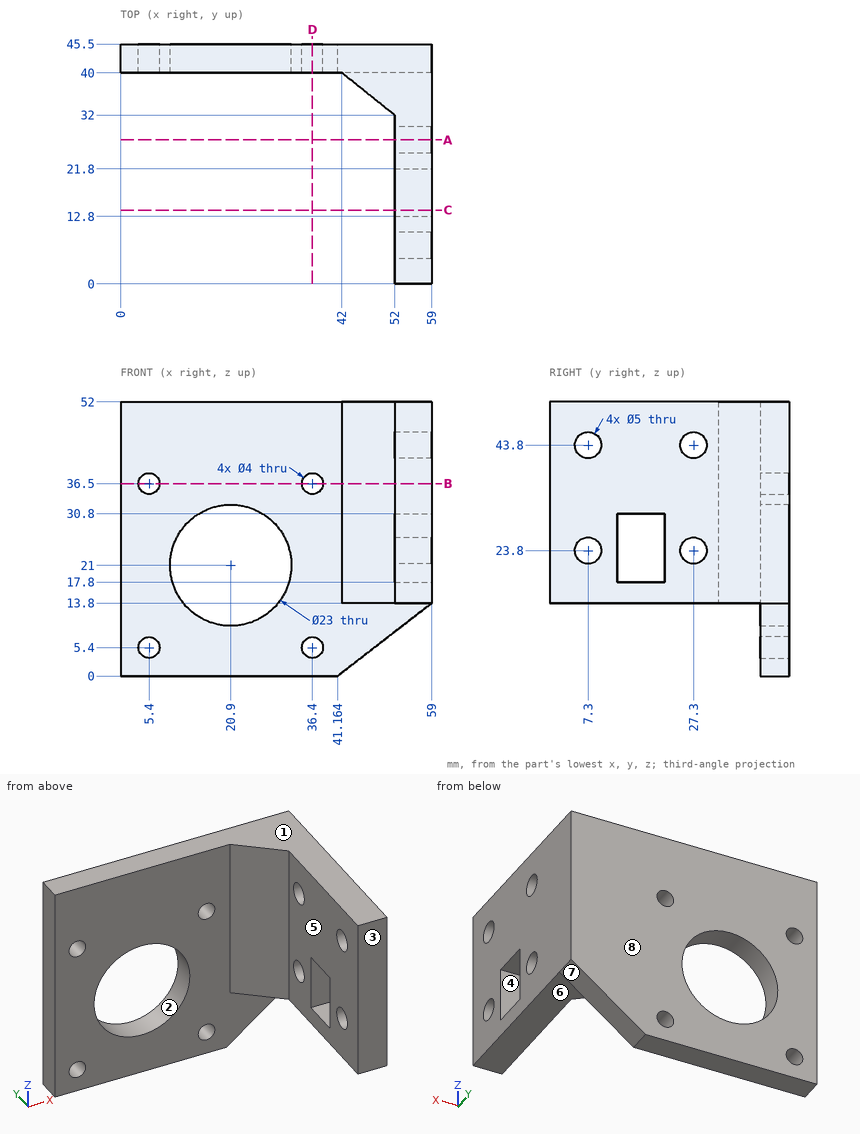
Study the drawing (mm; zero at the part's minimum x, y, z) and answer. A direction names the side the tool comes from. Coordinates: 2 decimals unless noted, no trailing zeros. Write each loop counter-clockwise with the first axis right and the second up, starting at its lowest first coordinate (ties: lowest second). Pieces come first, ordered by that corner, then holes.
Q1. Find the intervals of material crossed by line 1 (Z direction, x = 53, y = 7); line 2 (Y direction, x = 57, z = 43); line 3 (Y direction, x = 57.25, z = 43.8), in increasing order.
Q2. Which of the six approach directions +Z, -Z, +X, -X, +Y, -Y give full straight-line access (tool end or side, diameter ignored) to the marked faces 4, 5, 6, 7 and 8?
Q3. Determine the mould class of the marked faces 1, 2 and 3 for opening direction Z: released by +Z, released by -Z, zero draft, split by the parting line, or undercut.
Q4. A cutting plane is placed at B-B, the plane z = 36.5. Give the vertices of the cut face in (x, y).
Q5. A cutting plane is placed at C-C, the plane y = 14. Give the vertices of the cut face in (x, z), then the cut area to 3 significant figures.
Q6. A cutting plane is placed at D-D, the plane x = 36.4. Give the vertices of the cut face in (y, z), then the cut area to 3 significant figures.
Q7. Each of these flat-tipped pins is pushed along its axis until it touches: pin 1 Ø6.5 at (y, z) = (7.3, 23.8) entering from -X; pin 2 Ø5 at (y, z) = (11, 10) entering from -X; pin 3 Ø13.5 at (x, y) = (50.5, 25.5) entering from -Z; pin 4 Ø6.5 at (x, z) = (5.4, 36.5) entering from -Y. Where does it stop, or does it pass through?
Q8. A cutting plane is placed at A-A, the plane y = 27.3. Give the vertices of the cut face in (x, z).
Findings below:
1. line 1: z = 13.8 to 21.32, 26.28 to 41.32, 46.28 to 52
1. line 2: y = 0 to 4.93, 9.67 to 24.93, 29.67 to 45.5
1. line 3: y = 0 to 4.8, 9.8 to 24.8, 29.8 to 45.5
2. face 4: +X, -X
2. face 5: +Z, -Z, -X, -Y
2. face 6: -Z, +X, -X, -Y
2. face 7: -Z, +X, +Y, -Y
2. face 8: +Z, -Z, +X, -X, +Y
3. face 1: released by +Z
3. face 2: undercut
3. face 3: zero draft
4. outline: (0, 40) - (3.4, 40) - (3.4, 45.5) - (0, 45.5) - close; (7.4, 40) - (34.4, 40) - (34.4, 45.5) - (7.4, 45.5) - close; (38.4, 40) - (42, 40) - (52, 32) - (52, 0) - (59, 0) - (59, 45.5) - (38.4, 45.5) - close
5. outline: (52, 13.8) - (59, 13.8) - (59, 17.8) - (52, 17.8) - close; (52, 30.8) - (59, 30.8) - (59, 52) - (52, 52) - close
5. area: 176 mm2
6. outline: (40, 0) - (45.5, 0) - (45.5, 3.4) - (40, 3.4) - close; (40, 7.4) - (45.5, 7.4) - (45.5, 34.5) - (40, 34.5) - close; (40, 38.5) - (45.5, 38.5) - (45.5, 52) - (40, 52) - close
6. area: 242 mm2
7. pin 1: stops at x = 52
7. pin 2: passes through
7. pin 3: stops at z = 13.8
7. pin 4: stops at y = 40
8. outline: (52, 13.8) - (59, 13.8) - (59, 21.3) - (52, 21.3) - close; (52, 26.3) - (59, 26.3) - (59, 41.3) - (52, 41.3) - close; (52, 46.3) - (59, 46.3) - (59, 52) - (52, 52) - close
